Geometry check sheet. Reference: drawing and pictorial views, mm from the part's lowest x, y, z. A direction names the side the tool comes from. Give positions to 0.01 mm unless a question says otherwise; leave off trailing zeros. Loops run counter-clockwise (first coordinate to the right, second up) from the corner with the lowest first, then second, coordinate; pieces in that order, holes last. Notation, with made-up numbers: M 29.25,-0.75 L 79.25,-0.75 A14 cw 79.25,21.25 Z; hole C 9,-9.75 d6. An arc over 180 degrees is marked long. Put each result on its own line as item: value. Start each with the question number.
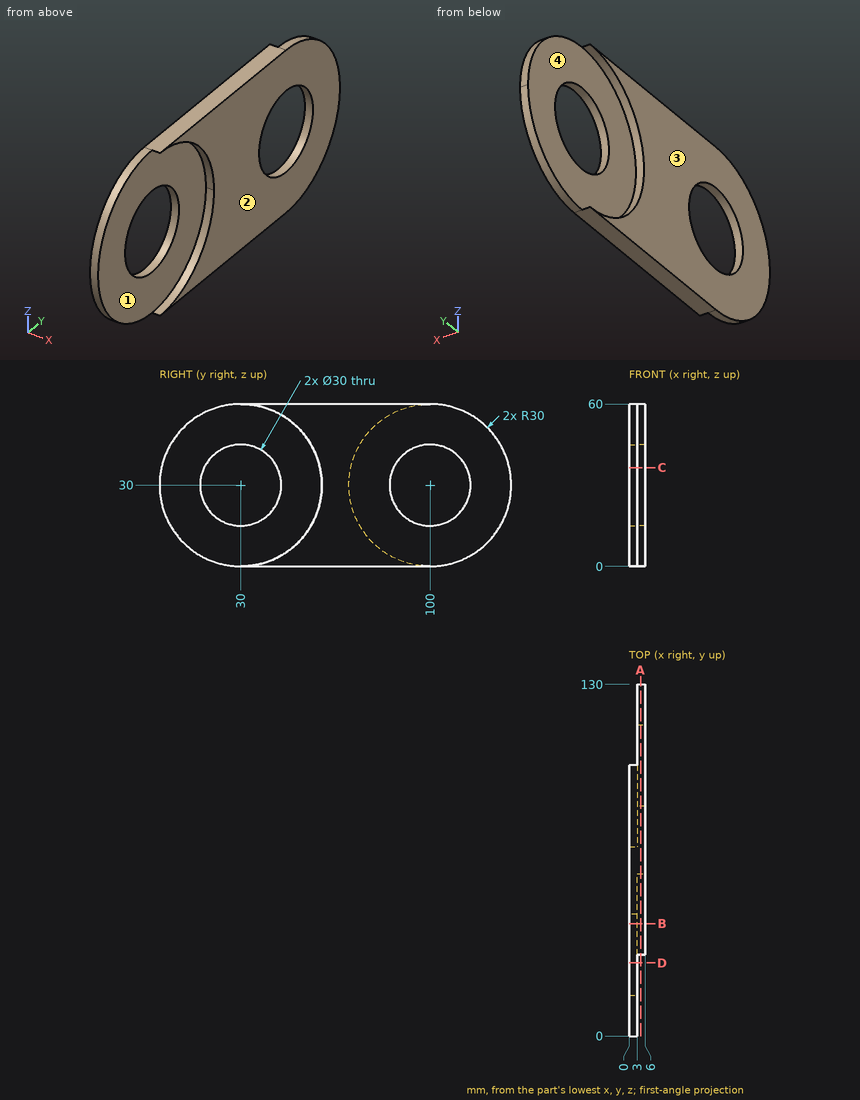
Q1. Section check C-C, the plane z = 36.5. Record the cut outline in (x, y), then the cut area to 3 significant figures.
Q2. Access from +Z, -Z, +X, -X, +Y, -Y to the whole of each face (thin tool, end or side, straight path). Record for the marked faces 3 and 4.
Q3. Thickness scan on line 1 along Z through (x, y) = (4.15, 100); line 2 along X through (y, z) = (114, 24); line 3 along Z through (x, y) = (5.6, 89). Record the ranges inside material, lowest first. Write a range as [from, to].
Q4. Mould release check, pull along Z, two halves, no side actions. Record for the marked faces 1 and 2: pulls with the +Z half, pulls with the -Z half, needs draft (parallel to the pull), parting line crosses it, or undercut.
Q5. Section check B-B, the plane y = 41.5. Record the cut outline in (x, z).
Q6. Section check A-A, the plane x = 4.2. Record the cut outline in (y, z).
Q7. Section check D-D, the plane y = 27. Record the cut outline in (x, z), then the cut area to 3 significant figures.
Q8. Depth check by flat-ended pin: P1, Ø2, axis at x = 0.5, z = 50, coming from the +Y side; P2, Ø3, axis at y = 97.5, z = 14.5, coming from the -X side; P3, Ø1.5, axis at x = 3, y = 29, coming from the -Z side. Enter the tip coordinate at first touch or a pass-through.
Found:
1. outline: M 0,0.71 L 3,0.71 L 3,16.48 L 0,16.48 Z; M 0,43.52 L 3,43.52 L 3,59.29 L 6,59.29 L 6,86.48 L 3,86.48 L 3,70.71 L 0,70.71 Z; M 3,113.52 L 6,113.52 L 6,129.29 L 3,129.29 Z
1. area: 258 mm^2
2. face 3: +Z, -Z, -X, +Y, -Y
2. face 4: -X, +Y
3. line 1: z = [0, 15], [45, 60]
3. line 2: x = [3, 6]
3. line 3: z = [0, 19.8], [40.2, 60]
4. face 1: undercut
4. face 2: needs draft
5. outline: M 0,0 L 6,0 L 6,2.29 L 3,2.29 L 3,20.37 L 0,20.37 Z; M 0,39.63 L 3,39.63 L 3,57.71 L 6,57.71 L 6,60 L 0,60 Z
6. outline: M 30,0 L 100,0 A30 ccw 130,30 A30 ccw 100,60 L 30,60 A30 cw 60,30 A30 cw Z; hole C 100,30 d30
7. outline: M 0,0.15 L 3,0.15 L 3,15.3 L 0,15.3 Z; M 0,44.7 L 3,44.7 L 3,59.85 L 0,59.85 Z
7. area: 90.9 mm^2
8. P1: stops at y = 78.58
8. P2: stops at x = 3
8. P3: stops at z = 0
